Design review of the part shown in the three views and the two pictorial views. Dimensions are in mm from the part's minimum x, y and z. A direction names the side the tool comes from. Coordinates: 2 decimals unless noted, no trailing zeros. Write each loop counter-clockwise with the first axis right and the second up, starting at its lowest first coordinate (ties: lowest second). Pieces come first, ordered by that corner, then holes.
Q1. For pin 1 Ø14 at (x, y) = (4.5, 6.5) entering from +Z (1 decimal); pin 2 Ø2 at (y, z) = (13, 26.5) entering from -X; pin 3 Ø1.5 at (x, y) = (23, 10.5) entering from +Z, all flat-tipped, find the tip position at first contact; note any pin that passes through.
Q2. For the marked faces 1 and 2, list the 3-axis set-ups (+Z, -Z, +X, -X, +Y, -Y) from which the entire face can be reached by the end or side of a thin tool; tool diameter is ignored.
Q3. Take a section at B-B, the plane x = 6.5. Write out the cut boundary in (y, z) (1 decimal).
Q4. For L1, parallel to Z at x = 9.5, y = 8.75 (1 decimal); L2, parallel to X at y = 1.25, z = 25; L3, parallel to Z at x = 22.5, y = 21 (1 decimal), list the stretches that pass through material, from the lowest coordinate up.
Q5. Take a section at C-C, the plane z = 18.5. Write out the cut boundary in (x, y), plus the area to 3 significant figures.
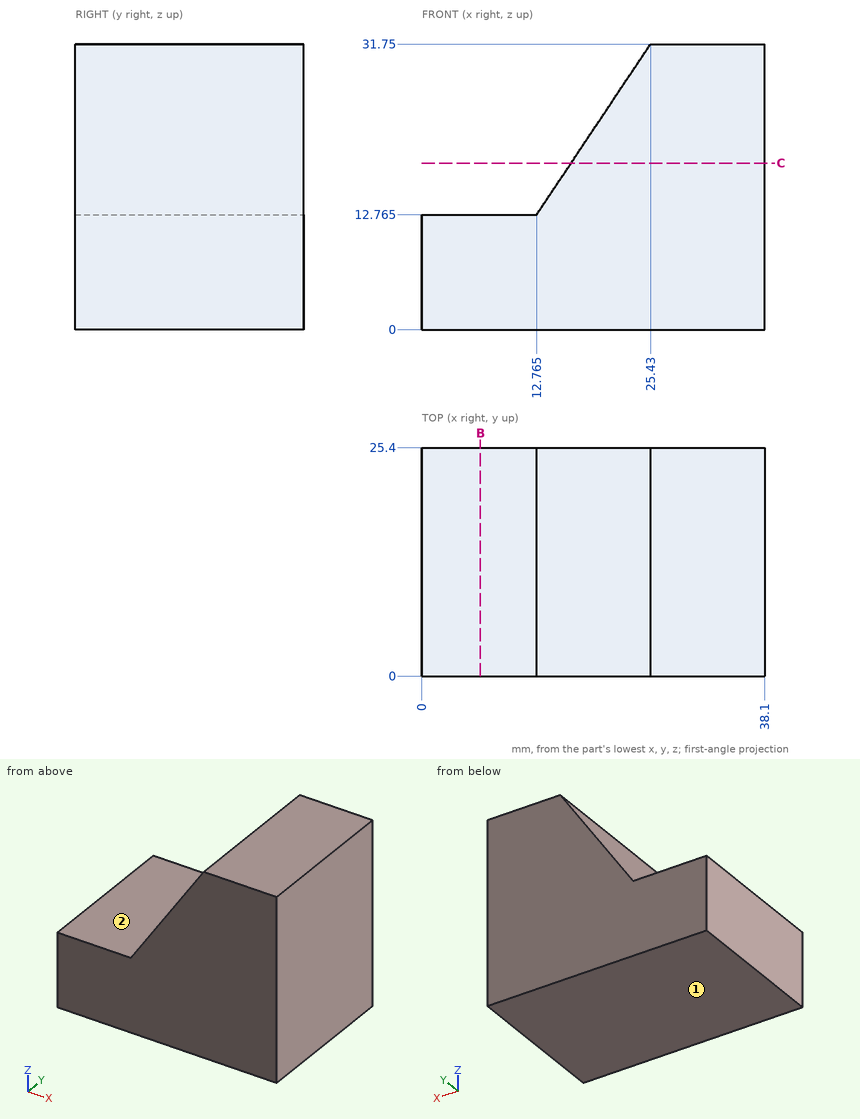
Responses:
1. pin 1: stops at z = 12.8
1. pin 2: stops at x = 21.26
1. pin 3: stops at z = 29.23
2. face 1: -Z, +X, -X, +Y, -Y
2. face 2: +Z, -X, +Y, -Y
3. outline: (0, 0) - (25.4, 0) - (25.4, 12.8) - (0, 12.8) - close
4. L1: z = 0 to 12.8
4. L2: x = 20.93 to 38.1
4. L3: z = 0 to 27.4
5. outline: (16.59, 0) - (38.1, 0) - (38.1, 25.4) - (16.59, 25.4) - close
5. area: 546 mm2
